from build123d import *

# Parameters (mm, degrees)
SKETCH2_W           = 12.4
SKETCH2_H           = 27.3
BOSS_EXTRUDE1_DEPTH = 81
SKETCH3_W           = 12.4
SKETCH3_H           = 1.2
BOSS_EXTRUDE2_DEPTH = 4.5
SKETCH6_W           = 12.4
SKETCH6_H           = 1.2
BOSS_EXTRUDE3_DEPTH = 4.5
SKETCH7_R           = 1
CUT_EXTRUDE2_DEPTH  = 4.5
SKETCH9_R           = 1
CUT_EXTRUDE3_DEPTH  = 1.2
SKETCH11_W          = 12.4
SKETCH11_H          = 32
CUT_EXTRUDE4_DEPTH  = 2
SKETCH12_R          = 1.5
CUT_EXTRUDE5_DEPTH  = 3
SKETCH13_W          = 14.8
SKETCH13_H          = 29.7
BOSS_EXTRUDE4_DEPTH = 1.2
EXTRUDE_THIN4_DEPTH = 27.3


with BuildPart() as part:
    # Sketch2 → Boss-Extrude1 (new body)
    with BuildSketch(Plane(origin=(0, 0, 16), x_dir=(-1, 0, 0), z_dir=(0, 0, -1))):
        Polygon((-1.710644683, 9.412349839), (10.689355317, 9.412349839), (11.889355317, 9.412349839), (11.889355317, -20.287650161), (-2.910644683, -20.287650161), (-2.910644683, 9.412349839), align=None)
        with Locations((4.489355317, -5.437650161)):
            Rectangle(SKETCH2_W, SKETCH2_H, mode=Mode.SUBTRACT)
    extrude(amount=-BOSS_EXTRUDE1_DEPTH)

    # Sketch3 → Boss-Extrude2 (add)
    with BuildSketch(Plane(origin=(0, 0, 20.5), x_dir=(-1, 0, 0), z_dir=(0, 0, -1))):
        with Locations((4.489355317, 1.512349839)):
            Rectangle(SKETCH3_W, SKETCH3_H)
    extrude(amount=BOSS_EXTRUDE2_DEPTH)

    # Sketch6 → Boss-Extrude3 (add)
    with BuildSketch(Plane.XY.offset(43.5)):
        with Locations((-4.489355317, 1.512349839)):
            Rectangle(SKETCH6_W, SKETCH6_H)
    extrude(amount=BOSS_EXTRUDE3_DEPTH)

    # Sketch7 → Cut-Extrude2 (cut)
    with BuildSketch(Plane(origin=(0, 2.112349839, 0), x_dir=(1, 0, 0), z_dir=(0, 1, 0))):
        with Locations(Location((-4.489355317, -46.25, 0), (0, 0, 270))):
            Circle(SKETCH7_R)
    extrude(amount=-CUT_EXTRUDE2_DEPTH, mode=Mode.SUBTRACT)

    # Sketch9 → Cut-Extrude3 (cut)
    with BuildSketch(Plane(origin=(0, 2.112349839, 0), x_dir=(1, 0, 0), z_dir=(0, 1, 0))):
        with Locations(Location((-4.489355317, -17.75, 0), (0, 0, 270))):
            Circle(SKETCH9_R)
    extrude(amount=-CUT_EXTRUDE3_DEPTH, mode=Mode.SUBTRACT)

    # Sketch11 → Cut-Extrude4 (cut)
    with BuildSketch(Plane(origin=(0, 9.412349839, 0), x_dir=(1, 0, 0), z_dir=(0, 1, 0))):
        with Locations((-4.489355317, -32)):
            Rectangle(SKETCH11_W, SKETCH11_H)
    extrude(amount=-CUT_EXTRUDE4_DEPTH, mode=Mode.SUBTRACT)

    # Sketch12 → Cut-Extrude5 (cut)
    with BuildSketch(Plane.XZ.offset(20.287650161)):
        with Locations((-4.489355317, 27)):
            Circle(SKETCH12_R)
    extrude(amount=-CUT_EXTRUDE5_DEPTH, mode=Mode.SUBTRACT)

    # Sketch13 → Boss-Extrude4 (add)
    with BuildSketch(Plane(origin=(0, 0, 16), x_dir=(-1, 0, 0), z_dir=(0, 0, -1))):
        with Locations((4.489355317, -5.437650161)):
            Rectangle(SKETCH13_W, SKETCH13_H)
    extrude(amount=BOSS_EXTRUDE4_DEPTH)

    # Sketch14 → Extrude-Thin4 (add)
    with BuildSketch(Plane.XZ.offset(-8.212349839)):
        Polygon((-11.186012312, 48.649869812), (2.450882677, 62.2867648), (2.648872575, 62.088774902), (-10.988022413, 48.451879913), align=None)
        Polygon((2.450882677, 48.896001763), (-11.245895089, 62.592779529), (-11.04790519, 62.790769427), (2.648872575, 49.093991662), align=None)
        Polygon((-11.186012312, 58.226694419), (2.450882677, 71.863589408), (2.648872575, 71.665599509), (-10.988022413, 58.02870452), align=None)
        Polygon((2.450882677, 58.47282637), (-11.245895089, 72.169604136), (-11.04790519, 72.367594035), (2.648872575, 58.670816269), align=None)
        Polygon((-11.186012312, 67.803519026), (2.450882677, 81.440414015), (2.648872575, 81.242424116), (-10.988022413, 67.605529127), align=None)
        Polygon((2.450882677, 68.049650977), (-11.245895089, 81.746428743), (-11.04790519, 81.944418642), (2.648872575, 68.247640876), align=None)
        Polygon((-11.186012312, 77.380343633), (2.450882677, 91.017238622), (2.648872575, 90.819248723), (-10.988022413, 77.182353735), align=None)
        Polygon((2.450882677, 77.626475585), (-11.245895089, 91.32325335), (-11.04790519, 91.521243249), (2.648872575, 77.824465483), align=None)
        Polygon((-10.82008194, 87.323098613), (-1.143180553, 97), (-0.945190654, 96.802010101), (-10.622092041, 87.125108714), align=None)
        Polygon((1.710644683, 87.943538186), (-7.345817131, 97), (-7.147827233, 97.197989899), (1.908634582, 88.141528084), align=None)
    extrude(amount=EXTRUDE_THIN4_DEPTH)


solid = part.part
Can you work these out from the model? Positions are in its coordinate system, mm. A direction names the side the tool comes from. Coordinates: 2 decimals unless noted, no trailing zeros. Write each loop counter-clockwise with the first axis right and the second up, starting at its lowest first coordinate (ties: lowest second). Pieces come first, ordered by that corner, then holes. Notation, with made-up numbers: (37.5, 76.5) - (96.5, 76.5) arc R19 cw to (96.5, 80.5) - close; hole circle Ø3 at (-1.5, 14). An arc over 180 degrees is marked (long way). Return JSON: item names as keys, results as strings. Group by question number.
Item 1: If we section it at A-A (z = 27): Write out the boundary of the cut face in (x, y).
Item 2: Please list where these lines run through material, in increasing order: probe 1 along X at (y, z) = (1.65, 46.25); probe 2 along Y at (x, z) = (-3.75, 44); probe 3 along Y at (x, z) = (-1, 60).
Item 3: If we section it at B-B (z = 42.5): Write out the boundary of the cut face in (x, y), then the cut area to 3 significant figures.
Item 4: If we section it at D-D (z = 17.75): Write out the boundary of the cut face in (x, y).
Item 5: I'm going to push flat-ended pins straight in: pin 1 Ø1.2 at (x, z) = (-4.49, 46.25) entering from +Y; pin 2 Ø8 at (x, y) = (-5, 7) entering from +Z; pin 3 Ø4 at (x, y) = (-5, -1.5) entering from +Z; pin 4 Ø4.5 at (x, y) = (-3.5, 1) entering from +Z. Where does each tip first touch, or does it pass through?
Item 6: Which directions (+Z, -Z, +X, -X, +Y, -Y) give clear straight access to the entire face, cutting with the end or side of a thin tool? Please do faces 1 (the face through (-4.685, -19.696, 28.487)), 2 (the face through (-4.189, 1.521, 47.204)), 3 (the face through (-10.689, -5, 94)), 4 (the face through (-6.31, -5.247, 72.284)).
Item 7: If we section it at C-C (y = -9.75): Count the separate pieces of the cut face and the enclosed holes in it, then the cut area to 3 significant figures.
Return value:
{
 "1": {"outline": "(-11.89, -20.29) - (-5.99, -20.29) - (-5.99, -19.09) - (-10.69, -19.09) - (-10.69, 9.41) - (-11.89, 9.41) - close; (-2.99, -20.29) - (2.91, -20.29) - (2.91, 9.41) - (1.71, 9.41) - (1.71, -19.09) - (-2.99, -19.09) - close"},
 "2": {"probe 1": "x = -11.89 to -5.49, -3.49 to 2.91", "probe 2": "y = -20.29 to -19.09, 0.91 to 2.11", "probe 3": "y = -20.29 to -19.09, 8.21 to 9.41"},
 "3": {"outline": "(-11.89, -20.29) - (2.91, -20.29) - (2.91, 9.41) - (1.71, 9.41) - (1.71, -19.09) - (-10.69, -19.09) - (-10.69, 9.41) - (-11.89, 9.41) - close", "area": "86.2 mm^2"},
 "4": {"outline": "(-11.89, -20.29) - (2.91, -20.29) - (2.91, 9.41) - (1.71, 9.41) - (1.71, 2.11) - (-3.49, 2.11) - (-3.49, 0.91) - (1.71, 0.91) - (1.71, -19.09) - (-10.69, -19.09) - (-10.69, 0.91) - (-5.49, 0.91) - (-5.49, 2.11) - (-10.69, 2.11) - (-10.69, 9.41) - (-11.89, 9.41) - close"},
 "5": {"pin 1": "stops at y = -19.09", "pin 2": "stops at z = 97.2", "pin 3": "stops at z = 97.05", "pin 4": "stops at z = 96.89"},
 "6": {"face 1": "+Y, -Y", "face 2": "+Y", "face 3": "+Z", "face 4": "none"},
 "7": {"separate pieces": "1", "enclosed holes": "21", "area": "258 mm^2"}
}
